Geometry: final body of the model. Coordinates: model frame, mm. Coordinates: 2 decimals unless noted, no trailing zeros. Loops run counter-clockwise (first coordinate to the right, second up) from the corner with the lowest first, then second, coordinate; pieces in that order, holes last. Notation, with made-up numbers: (7.5, -27.75) - (59.5, -27.75) arc R10 ccw to (59.5, -12.75) - close; hole circle Ø2 at (88.25, 50.5). An arc over 180 degrees is marked (long way). Answer in a Markdown table with one row per item.
from build123d import *

# Parameters (mm, degrees)
SKETCH_W        = 50
SKETCH_H        = 118
PAD_DEPTH       = 3
SKETCH001_W     = 50
SKETCH001_H     = 3
PAD001_DEPTH    = 3
SKETCH002_W     = 44
SKETCH002_H     = 78
SKETCH002_H_2   = 27
POCKET_DEPTH    = 3
CHAMFER_SIZE    = 2
CHAMFER001_SIZE = 1


with BuildPart() as part:
    # Sketch → Pad (new body)
    with BuildSketch(Plane.XY):
        with Locations((25, 59)):
            Rectangle(SKETCH_W, SKETCH_H)
    extrude(amount=PAD_DEPTH)

    # Sketch001 (on Face6 of Pad) → Pad001 (join)
    with BuildSketch(Plane.XY.offset(3)):
        with Locations((25, 1.5)):
            Rectangle(SKETCH001_W, SKETCH001_H)
    extrude(amount=PAD001_DEPTH)

    # Sketch002 (on Face3 of Pad001) → Pocket (cut)
    with BuildSketch(Plane.XY.offset(3)):
        with Locations((25, 44)):
            Rectangle(SKETCH002_W, SKETCH002_H)
        with Locations((25, 101.5)):
            Rectangle(SKETCH002_W, SKETCH002_H_2)
    extrude(amount=-POCKET_DEPTH, mode=Mode.SUBTRACT)

    # Chamfer
    chamfer_edges = [part.edges().sort_by_distance(p)[0] for p in [
        (25, 115, 3),
    ]]
    chamfer(chamfer_edges, length=CHAMFER_SIZE)

    # Chamfer001
    chamfer001_edges = [part.edges().sort_by_distance(p)[0] for p in [
        (25, 5, 3),
    ]]
    chamfer(chamfer001_edges, length=CHAMFER001_SIZE)


solid = part.part
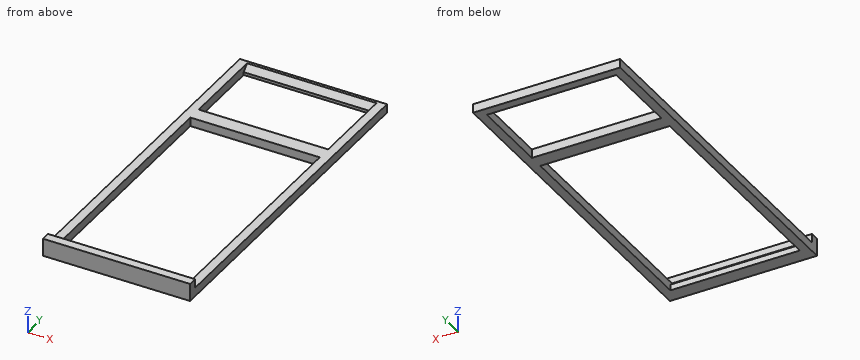
(1) Cut plane C-C on z = 4.25. Output: boundary loops of the cut face in (x, y), then the cut area to 3 significant figures.
Verdict:
| item | result |
|---|---|
| outline | (0, 0) - (50, 0) - (50, 3) - (0, 3) - close |
| area | 150 mm² |
(2) Cut plane B-B on y = 18. Output: boundary loops of the cut face in (x, z).
Verdict:
| item | result |
|---|---|
| outline | (0, 0) - (3, 0) - (3, 3) - (0, 3) - close; (47, 0) - (50, 0) - (50, 3) - (47, 3) - close |
(3) Cut plane A-A on x = 27.5. Output: boundary loops of the cut face in (y, z).
Verdict:
| item | result |
|---|---|
| outline | (0, 0) - (5, 0) - (5, 2) - (4, 3) - (3, 3) - (3, 6) - (0, 6) - close; (83, 0) - (88, 0) - (88, 3) - (83, 3) - close; (115, 0) - (118, 0) - (118, 3) - (117, 3) - (115, 1) - close |
(4) Ray query, probe 1 along Y at (x, z) = (36.5, 0.35); probe 2 along X at (y, z) = (107, 0.45); probe 3 along Y at (x, z) = (38.5, 1.3). Return the intervals inside material, ascending.
Verdict:
| item | result |
|---|---|
| probe 1 | y = 0 to 5, 83 to 88, 115 to 118 |
| probe 2 | x = 0 to 3, 47 to 50 |
| probe 3 | y = 0 to 5, 83 to 88, 115.3 to 118 |
(5) First-contact query: pin 1 Ø3 at (x, z) = (33, 5.5) entering from +Y. Flat tip, straight axial feed; report the tip coordinate or a pass-through.
Verdict:
| item | result |
|---|---|
| pin 1 | stops at y = 3 |
